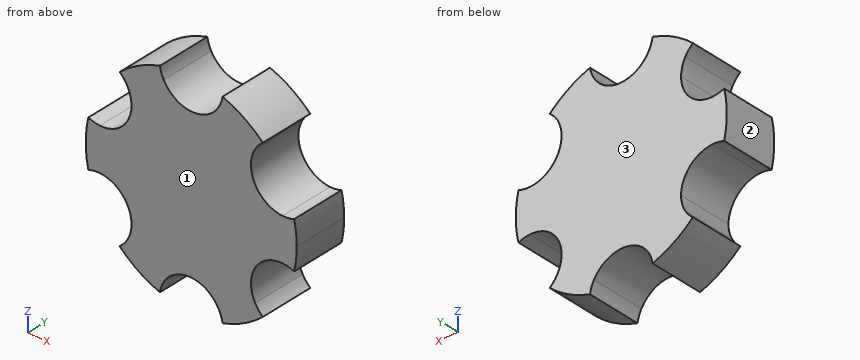
```python
from build123d import *

# Parameters (mm, degrees)
F2_DEPTH = 10


with BuildPart() as f2:
    # F1 (on offset) → F2 (new body)
    with BuildSketch(Plane.XZ.offset(-20)):
        with BuildLine():
            ThreePointArc((12.124355653, 13), (12.7707828093, 13.9115214431), (13.5750272223, 14.6873631369))
            ThreePointArc((13.5750272223, 14.6873631369), (10, 17.3205080757), (5.93211598, 19.1))
            ThreePointArc((5.93211598, 19.1), (5.6623395704, 18.0155830606), (5.1961524227, 17))
            Line((5.1961524227, 17), (12.124355653, 13))
        make_face()
        with BuildLine():
            ThreePointArc((19.5071432023, -4.4126368631), (19.8764039007, -2.2200378324), (20, 0))
            ThreePointArc((20, 0), (19.8764039007, 2.2200378324), (19.5071432023, 4.4126368631))
            ThreePointArc((19.5071432023, 4.4126368631), (18.4331223797, 4.1040616175), (17.3205080757, 4))
            Line((17.3205080757, 4), (17.3205080757, -4))
            ThreePointArc((17.3205080757, -4), (18.4331223797, -4.1040616175), (19.5071432023, -4.4126368631))
        make_face()
        with BuildLine():
            Line((17.3205080757, -4), (17.3205080757, 4))
            ThreePointArc((17.3205080757, 4), (12.124355653, 7), (12.124355653, 13))
            Line((12.124355653, 13), (5.1961524227, 17))
            ThreePointArc((5.1961524227, 17), (0, 14), (-5.1961524227, 17))
            Line((-5.1961524227, 17), (-12.124355653, 13))
            ThreePointArc((-12.124355653, 13), (-11.524953118, 11.5529142706), (-11.3205080757, 10))
            ThreePointArc((-11.3205080757, 10), (-13.0778673886, 5.7573593129), (-17.3205080757, 4))
            Line((-17.3205080757, 4), (-17.3205080757, -4))
            ThreePointArc((-17.3205080757, -4), (-13.0778673886, -5.7573593129), (-11.3205080757, -10))
            ThreePointArc((-11.3205080757, -10), (-11.524953118, -11.5529142706), (-12.124355653, -13))
            Line((-12.124355653, -13), (-5.1961524227, -17))
            ThreePointArc((-5.1961524227, -17), (0, -14), (5.1961524227, -17))
            Line((5.1961524227, -17), (12.124355653, -13))
            ThreePointArc((12.124355653, -13), (12.124355653, -7), (17.3205080757, -4))
        make_face()
        with BuildLine():
            ThreePointArc((5.93211598, -19.1), (10, -17.3205080757), (13.5750272223, -14.6873631369))
            ThreePointArc((13.5750272223, -14.6873631369), (12.7707828093, -13.9115214431), (12.124355653, -13))
            Line((12.124355653, -13), (5.1961524227, -17))
            ThreePointArc((5.1961524227, -17), (5.6623395704, -18.0155830606), (5.93211598, -19.1))
        make_face()
        with BuildLine():
            ThreePointArc((-5.93211598, -19.1), (-5.6623395704, -18.0155830606), (-5.1961524227, -17))
            Line((-5.1961524227, -17), (-12.124355653, -13))
            ThreePointArc((-12.124355653, -13), (-12.7707828093, -13.9115214431), (-13.5750272223, -14.6873631369))
            ThreePointArc((-13.5750272223, -14.6873631369), (-10, -17.3205080757), (-5.93211598, -19.1))
        make_face()
        with BuildLine():
            Line((-12.124355653, 13), (-5.1961524227, 17))
            ThreePointArc((-5.1961524227, 17), (-5.6623395704, 18.0155830606), (-5.93211598, 19.1))
            ThreePointArc((-5.93211598, 19.1), (-10, 17.3205080757), (-13.5750272223, 14.6873631369))
            ThreePointArc((-13.5750272223, 14.6873631369), (-12.7707828093, 13.9115214431), (-12.124355653, 13))
        make_face()
        with BuildLine():
            ThreePointArc((-17.3205080757, 4), (-18.4331223797, 4.1040616175), (-19.5071432023, 4.4126368631))
            ThreePointArc((-19.5071432023, 4.4126368631), (-20, 0), (-19.5071432023, -4.4126368631))
            ThreePointArc((-19.5071432023, -4.4126368631), (-18.4331223797, -4.1040616175), (-17.3205080757, -4))
            Line((-17.3205080757, -4), (-17.3205080757, 4))
        make_face()
    extrude(amount=F2_DEPTH)


solid = f2.part
```
Model file for the job. Use its own axes, mm. Face numbers are marked on the shaded views. Coordinates: 2 decimals unless noted, no trailing zeros. Loops run counter-clockwise (first coordinate to the right, second up) from the corner with the lowest first, then second, coordinate; pieces in that order, holes last. Notation, with made-up numbers: (3, 82.25) - (27, 82.25) arc R15 ccw to (27, 95.25) - close; hole circle Ø5 at (-12.75, 32.25). An arc over 180 degrees is marked (long way). Write item = value, one per line. Start each with the question number.
Item 1: Saw through at A-A, the plane y = 10.5. List the corners of the cut face in (x, z).
Item 2: Drop flat-ended pins along their axis: pin 1 Ø3 at (y, z) = (17, 1) entering from -X; pin 2 Ø1.5 at (y, z) = (14, 5) entering from +X; pin 3 Ø2 at (x, y) = (8, 15) entering from -Z (3 decimals). Give the stop position or say it passes through.
Item 3: Saw through at B-B, the plane x = 10. List the corners of the cut face in (y, z), then the cut area to 3 significant figures.
Item 4: Pull direction Y, two halves, no side cores. Call the marked faces 1, 2 and 3: +Y half, -Y half, draft (parallel to the pull), parting line (faces both ways), or undercut.
Item 5: Saw through at C-C, the plane z = -5.5. List the corners of the cut face in (x, y), then the cut area to 3 significant figures.
Item 6: Wall check: probe 1 along X at (y, z) = (14.5, 10); probe 2 along X at (y, z) = (17.25, -7); probe 3 along Z at (x, y) = (-10, 15.5). Give the ranges that are in metal, low to high. Write a range as [from, to].
Answers:
q1.outline = (-19.51, -4.41) arc R6 cw to (-13.58, -14.69) arc R20 ccw to (-5.93, -19.1) arc R6 cw to (5.93, -19.1) arc R20 ccw to (13.58, -14.69) arc R6 cw to (19.51, -4.41) arc R20 ccw to (19.51, 4.41) arc R6 cw to (13.58, 14.69) arc R20 ccw to (5.93, 19.1) arc R6 cw to (-5.93, 19.1) arc R20 ccw to (-13.58, 14.69) arc R6 cw to (-19.51, 4.41) arc R20 ccw to start
q2.pin_1 = -20
q2.pin_2 = 19.54
q2.pin_3 = -18.735
q3.outline = (10, -17.32) - (20, -17.32) - (20, 17.32) - (10, 17.32) - close
q3.area = 346 mm2
q4.face_1 = -Y half
q4.face_2 = draft
q4.face_3 = +Y half
q5.outline = (-13.35, 10) - (13.35, 10) - (13.35, 20) - (-13.35, 20) - close
q5.area = 267 mm2
q6.probe_1 = [-11.32, 11.32]
q6.probe_2 = [-12.12, 12.12]
q6.probe_3 = [-17.32, 17.32]
